Part model, mm, in its own coordinate system. Face numbers are marked on the shaded views. A direction names the side the tool comes from. Coordinates: 2 decimals unless noted, no trailing zeros. Loops run counter-clockwise (first coordinate to the right, second up) from the corner with the lowest first, then second, coordinate; pieces in that order, holes last. Notation, with made-up numbers: (-34, 44.5) - (4, 44.5) arc R11 ccw to (4, 49.5) - close; hole circle Ø5 at (56.25, -39.5). An arc over 180 degrees is marked (long way). Use a Markdown table: item, result. Add a question column.
1. Band-saw the part on D-D, the plane x = 20. Give the cut face in (y, z), plus the area to 3 significant figures.
2. Band-saw the part on B-B, the plane x = -4. Give the cut face in (y, z).
3. Band-saw the part on C-C, the plane z = -3. Give the cut face in (x, y), plus the area to 3 significant figures.
4. Band-saw the part on A-A, the plane y = 5.5. Give the cut face in (x, z), plus the area to 3 significant figures.
5. Drop flat-ended pins along their axis: pin 1 (1.5 mm diameter, centred on x = 11, z = -6.5, fed in from +Y); pin 2 (1 mm diameter, centred on y = 6.5, z = 13.5, fed in from -X); pin 3 (1.6 mm diameter, centred on y = 5, z = 9, fed in from -X). Give the stop position or say it passes through.
6. 3-axis set-ups, long thin cutter, end or side, ignore diameter. For the marked faces 1, 2 and 3: which of +Z, -Z, +X, -X, +Y, -Y reach the whole face in a straight line?
7. Wall check: probe 1 along X at (y, z) = (0.25, 13); probe 2 along Y at (x, z) = (-13, -5); probe 3 along X at (y, z) = (7.5, 16.5). Give the ranges that are in metal, low to high. Write a range as [from, to].
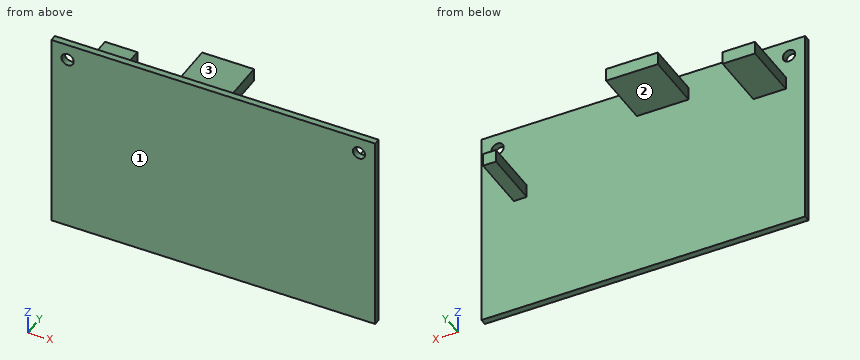
from build123d import *

# Parameters (mm, degrees)
BOSS_EXTRU_7_DEPTH      = 9
BOSS_EXTRU_7_DEPTH_BACK = 1
ESQUISSE1_W             = 8
ESQUISSE1_H             = 2
BOSS_EXTRU_8_DEPTH      = 9
BOSS_EXTRU_8_DEPTH_BACK = 1
ESQUISSE1_10_W          = 5
ESQUISSE1_10_H          = 2
BOSS_EXTRU_9_DEPTH      = 9
BOSS_EXTRU_9_DEPTH_BACK = 1
ESQUISSE1_11_W          = 2
ESQUISSE1_11_H          = 2
ESQUISSE1_12_W          = 50
ESQUISSE1_12_H          = 31
ESQUISSE1_12_R          = 0.95
ESQUISSE1_12_W_2        = 5
ESQUISSE1_12_H_2        = 2
ESQUISSE1_12_W_3        = 8
ESQUISSE1_12_W_4        = 2
BOSS_EXTRU_10_DEPTH     = 1


with BuildPart() as part:
    # Esquisse1 → Boss.-Extru.7 (new, two sides: drawn at the far end of the back side and taken through both)
    with BuildSketch(Plane(origin=(0, 0, 0), x_dir=(1, 0, 0), z_dir=(0, 1, 0)).offset(-BOSS_EXTRU_7_DEPTH_BACK)):
        with Locations((-0.479564033, -17.121253406)):
            Rectangle(ESQUISSE1_W, ESQUISSE1_H)
    extrude(amount=BOSS_EXTRU_7_DEPTH + BOSS_EXTRU_7_DEPTH_BACK)



with BuildPart() as body_2:
    # Esquisse1_10 → Boss.-Extru.8 (new, two sides: drawn at the far end of the back side and taken through both)
    with BuildSketch(Plane(origin=(0, 0, 0), x_dir=(1, 0, 0), z_dir=(0, 1, 0)).offset(-BOSS_EXTRU_8_DEPTH_BACK)):
        with Locations((-16.979564033, -13.621253406)):
            Rectangle(ESQUISSE1_10_W, ESQUISSE1_10_H)
    extrude(amount=BOSS_EXTRU_8_DEPTH + BOSS_EXTRU_8_DEPTH_BACK)


with BuildPart() as body_3:
    # Esquisse1_11 → Boss.-Extru.9 (new, two sides: drawn at the far end of the back side and taken through both)
    with BuildSketch(Plane(origin=(0, 0, 0), x_dir=(1, 0, 0), z_dir=(0, 1, 0)).offset(-BOSS_EXTRU_9_DEPTH_BACK)):
        with Locations((21.520435967, -9.286103542)):
            Rectangle(ESQUISSE1_11_W, ESQUISSE1_11_H)
    extrude(amount=BOSS_EXTRU_9_DEPTH + BOSS_EXTRU_9_DEPTH_BACK)


with BuildPart() as part_1:
    add(part.part)

    add(body_2.part)  # Boss.-Extru.10 merges body 2

    add(body_3.part)  # Boss.-Extru.10 merges body 3
    # Esquisse1_12 → Boss.-Extru.10 (add)
    with BuildSketch(Plane(origin=(0, 0, 0), x_dir=(1, 0, 0), z_dir=(0, 1, 0))):
        with Locations((2.520435967, -5.121253406)):
            Rectangle(ESQUISSE1_12_W, ESQUISSE1_12_H)
        with Locations(Location((-19.979564033, -18.121253406, 0), (0, 0, 270))):
            Circle(ESQUISSE1_12_R, mode=Mode.SUBTRACT)
        with Locations(Location((25.020435967, -18.121253406, 0), (0, 0, 270))):
            Circle(ESQUISSE1_12_R, mode=Mode.SUBTRACT)
        with Locations((-16.979564033, -13.621253406)):
            Rectangle(ESQUISSE1_12_W_2, ESQUISSE1_12_H_2, mode=Mode.SUBTRACT)
        with Locations((-0.479564033, -17.121253406)):
            Rectangle(ESQUISSE1_12_W_3, ESQUISSE1_12_H_2, mode=Mode.SUBTRACT)
        with Locations((21.520435967, -9.286103542)):
            Rectangle(ESQUISSE1_12_W_4, ESQUISSE1_12_H_2, mode=Mode.SUBTRACT)
    extrude(amount=-BOSS_EXTRU_10_DEPTH)


solid = part_1.part
Geometry check:
| question | item | result |
|---|---|---|
| 1 | outline | (-1, -10.38) - (0, -10.38) - (0, 20.62) - (-1, 20.62) - close |
| 1 | area | 31.0 mm^2 |
| 2 | outline | (-1, -10.38) - (0, -10.38) - (0, 16.12) - (9, 16.12) - (9, 18.12) - (0, 18.12) - (0, 20.62) - (-1, 20.62) - close |
| 3 | outline | (-22.48, -1) - (27.52, -1) - (27.52, 0) - (-22.48, 0) - close |
| 3 | area | 50.0 mm^2 |
| 4 | outline | (-19.48, 12.62) - (-14.48, 12.62) - (-14.48, 14.62) - (-19.48, 14.62) - close; (-4.48, 16.12) - (3.52, 16.12) - (3.52, 18.12) - (-4.48, 18.12) - close; (20.52, 8.29) - (22.52, 8.29) - (22.52, 10.29) - (20.52, 10.29) - close |
| 4 | area | 30.0 mm^2 |
| 5 | pin 1 | stops at y = 0 |
| 5 | pin 2 | stops at x = -19.48 |
| 5 | pin 3 | stops at x = 20.52 |
| 6 | face 1 | +Z, -Z, +X, -X, -Y |
| 6 | face 2 | -Z, +X, -X, +Y |
| 6 | face 3 | +Z, +X, -X, +Y |
| 7 | probe 1 | x = [-19.48, -14.48] |
| 7 | probe 2 | y = [-1, 0] |
| 7 | probe 3 | x = [-4.48, 3.52] |
